Work out the finished part from the listing and answer in its coordinate system (mm). Round coordinates to 2 decimals unless told otherwise and drop trailing zeros. Loops run counter-clockwise (first coordinate to the right, second up) from the corner with the lowest first, then second, coordinate; pieces in that order, holes last.
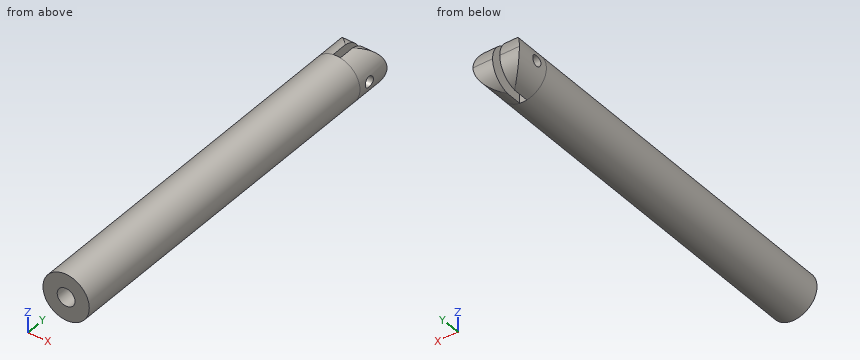
```python
from build123d import *

# Parameters (mm, degrees)
SKETCH1_R               = 6.5
SKETCH1_R_2             = 2.5
BOSS_EXTRUDE1_DEPTH     = 100
SKETCH2_R               = 6.5
BOSS_EXTRUDE2_DEPTH     = 10
BOSS_EXTRUDE3_DEPTH     = 10
CUT_EXTRUDE2_DEPTH      = 7.5
CUT_EXTRUDE2_DEPTH_BACK = 7.5
SKETCH5_R               = 1.5
CUT_EXTRUDE3_DEPTH      = 8.5
CUT_EXTRUDE3_DEPTH_BACK = 6.5


with BuildPart() as part:
    # Sketch1 → Boss-Extrude1 (new body)
    with BuildSketch(Plane(origin=(0, 0, 0), x_dir=(1, 0, 0), z_dir=(0, 1, 0))):
        Circle(SKETCH1_R)
        Circle(SKETCH1_R_2, mode=Mode.SUBTRACT)
    extrude(amount=BOSS_EXTRUDE1_DEPTH)

    # Sketch2 → Boss-Extrude2 (add)
    with BuildSketch(Plane(origin=(0, 100, 0), x_dir=(1, 0, 0), z_dir=(0, 1, 0))):
        Circle(SKETCH2_R)
    extrude(amount=-BOSS_EXTRUDE2_DEPTH)

    # Sketch3 → Boss-Extrude3 (add)
    with BuildSketch(Plane(origin=(0, 100, 0), x_dir=(1, 0, 0), z_dir=(0, 1, 0))):
        with BuildLine():
            Line((-1, -6.422616), (-1, 6.422616))
            ThreePointArc((-1, 6.422616), (-6.5, 0), (-1, -6.422616))
        make_face()
        with BuildLine():
            Line((1, -6.422616), (1, 6.422616))
            ThreePointArc((1, 6.422616), (6.5, 0), (1, -6.422616))
        make_face()
    extrude(amount=BOSS_EXTRUDE3_DEPTH)

    # Sketch4 → Cut-Extrude2 (cut, two sides)
    with BuildSketch(Plane(origin=(0, 0, 0), x_dir=(0, 0, -1), z_dir=(1, 0, 0))) as cut_extrude2_sk:
        with BuildLine():
            ThreePointArc((0, 110), (4.541154, 108.150583), (6.498158, 103.654745))
            Line((6.498158, 103.654745), (6.422616, 110))
            Line((6.422616, 110), (0, 110))
        make_face()
        with BuildLine():
            Line((-6.422616, 110), (-6.498158, 103.654745))
            ThreePointArc((-6.498158, 103.654745), (-4.541154, 108.150583), (0, 110))
            Line((0, 110), (-6.422616, 110))
        make_face()
    extrude(amount=CUT_EXTRUDE2_DEPTH, mode=Mode.SUBTRACT)
    extrude(cut_extrude2_sk.sketch, amount=-CUT_EXTRUDE2_DEPTH_BACK, mode=Mode.SUBTRACT)

    # Sketch5 → Cut-Extrude3 (cut, two sides)
    with BuildSketch(Plane.ZY.offset(-1)) as cut_extrude3_sk:
        with Locations((0, 103.5)):
            Circle(SKETCH5_R)
    extrude(amount=CUT_EXTRUDE3_DEPTH, mode=Mode.SUBTRACT)
    extrude(cut_extrude3_sk.sketch, amount=-CUT_EXTRUDE3_DEPTH_BACK, mode=Mode.SUBTRACT)


solid = part.part
```
1. Given pin 1 (6 mm diameter, centred on x = 5, z = 1.5, fed in from +Y); pin 2 (1.6 mm diameter, centred on x = 0, z = 2, fed in from +Y); pin 3 (1 mm diameter, centred on x = -4.5, y = 69, fed in from +Z); pin 4 (3 mm diameter, centred on y = 104.5, z = -2, fed in from +X), each flat-ended and moving along its own axis, determine where each tip first touches the part or whether it passes through.
Answer key:
pin 1: stops at y = 110
pin 2: stops at y = 100
pin 3: stops at z = 5.12
pin 4: stops at x = 6.48
2. Find section C-C (z = -3.75). Write down the section's boundary in (x, y), then the cut area to 3 significant figures.
Answer key:
outline: (-5.31, 0) - (5.31, 0) - (5.31, 108.81) - (1, 108.81) - (1, 100) - (-1, 100) - (-1, 108.81) - (-5.31, 108.81) - close
area: 1,140 mm2
3. Find section B-B (x = 0). Write down the section's boundary in (y, z), then the cut area to 3 significant figures.
Answer key:
outline: (0, -6.5) - (100, -6.5) - (100, 6.5) - (0, 6.5) - (0, 2.5) - (90, 2.5) - (90, -2.5) - (0, -2.5) - close
area: 850 mm2
4. Find section D-D (y = 103.5). Write down the section's boundary in (x, z), then the cut area to 3 significant figures.
Answer key:
outline: (-6.32, -1.5) arc R6.5 ccw to (-1, -6.42) - (-1, -1.5) - close; (-6.32, 1.5) - (-1, 1.5) - (-1, 6.42) arc R6.5 ccw to start; (1, -6.42) arc R6.5 ccw to (6.32, -1.5) - (1, -1.5) - close; (1, 1.5) - (6.32, 1.5) arc R6.5 ccw to (1, 6.42) - close
area: 74.2 mm2
5. Consider probe 1 along Y at (x, z) = (3.1, 0); probe 2 along Z at (x, y) = (0, 76.5). Determine where each line is inside the solid, lowest interval first.
Answer key:
probe 1: y = 0 to 102, 105 to 110
probe 2: z = -6.5 to -2.5, 2.5 to 6.5
6. Find section A-A (y = 73.5). Write down the section's boundary in (x, z), then the cut area to 3 significant figures.
Answer key:
outline: circle Ø13 at (0, 0); hole circle Ø5 at (0, 0)
area: 113 mm2
